Design review of the part built by this model. Coordinates are the model's own, in mm. A direction names the side the tool comes from. Coordinates: 2 decimals unless noted, no trailing zeros. Loops run counter-clockwise (first coordinate to the right, second up) from the corner with the lowest first, then second, coordinate; pieces in that order, holes last. Notation, with made-up numbers: (65.5, -21.5) - (75.5, -21.5) arc R25 cw to (75.5, 6.5) - close; hole circle Ø11 at (-21, 89). An arc over 180 degrees is marked (long way). Use one line per item in the form item = value. Start each with the question number.
(1) The part is to be moulded in two halves that separate along Y. For faces 1 (the face through (0, -10, 9)), 2 (the face through (-35, 65, 9)), 3 (the face through (-20, 25, 9)), say which applies: pulls with the +Y half, pulls with the -Y half, needs draft (parallel to the pull), parting line crosses it, or undercut.
(2) Add section C-C (z = 11). State the section outline as (x, y) points.
(3) Tool access review of faces 4 (the face through (-15, 67, 18)), 5 (the face through (10, 41, 9)): name each direction out of +Z, -Z, +X, -X, +Y, -Y from which nothing blocks a thin tool from reaching the whole face with its end or side.
(4) Add section A-A (x = 0). State the section outline as (y, z) points, plus the area to 3 significant figures.
(5) Add section B-B (y = 56). State the section outline as (x, z) points.
(6) For L1, parallel to X at y = 49, z = 15; L2, parallel to Y at x = -7.5, z = 16.75; L3, parallel to Y at x = 5.5, z = 7.5, list the stretches that pass through material, from the lowest coordinate up.
(7) Clearance check with flat-ended pins moving along their axes: pin 1 Ø3 at (x, z) = (-12, 8) entering from -Y; pin 2 Ø10 at (x, y) = (-3.5, 73) entering from -Z; pin 3 Ø9 at (y, z) = (38.5, 10.5) entering from -X. State where each tip first meets the part, or that it passes through.
Autodesk Inventor part; units mm, degrees
ref_plane "YZ Plane" through (0, 0, 0) normal (1, 0, 0) x (0, 1, 0)
ref_plane "XZ Plane" through (0, 0, 0) normal (0, 1, 0) x (-1, 0, 0)
ref_plane "XY Plane" through (0, 0, 0) normal (0, 0, 1) x (1, 0, 0)
sketch "Sketch1" plane through (0, 0, 0) normal (0, 0, 1) x (1, 0, 0)
  line L0 (0, 0) -> (0, 80) construction
  line L1 (0, 80) -> (10, 80) construction
  line L2 (0, 80) -> (-10, 80) construction
  line L3 (-10, 80) -> (10, 80)
  line L4 (10, 80) -> (10, 0)
  line L5 (-10, 80) -> (-10, 0)
  arc A0 (-10, 0) -> (10, 0) centre (0, 0) ccw
  line L6 (10, 0) -> (20, 0) construction
  line L7 (20, 0) -> (20, 120)
  line L8 (20, 120) -> (-50, 120)
  line L9 (-50, 120) -> (-50, 80)
  line L10 (-50, 120) -> (-20, 120) construction
  arc A1 (-20, 0) -> (20, 0) centre (0, 0) ccw
  line L11 (-20, 0) -> (-20, 50)
  line L12 (-20, 50) -> (-50, 80)
  dimension "d0" = 80
  dimension "d3" = 10
  dimension "d4" = 120
  dimension "d5" = 70
  dimension "d6" = 40
  dimension "d7" = 30
  dimension "d8" = 20
  dimension "d9" = 50
extrude "Extrusion1" add sketch "Sketch1" along normal blind 18
properties part number "guide_3DPrint"
Computed values:
q1.face_1 = undercut
q1.face_2 = pulls with the -Y half
q1.face_3 = needs draft
q2.outline = (-50, 80) - (-20, 50) - (-20, 0) arc R20 ccw to (20, 0) - (20, 120) - (-50, 120) - close; hole (-10, 0) arc R10 ccw to (10, 0) - (10, 80) - (-10, 80) - close
q3.face_4 = +Z, +X, -X, +Y, -Y
q3.face_5 = +Z, -Z
q4.outline = (-20, 0) - (-10, 0) - (-10, 18) - (-20, 18) - close; (80, 0) - (120, 0) - (120, 18) - (80, 18) - close
q4.area = 900 mm^2
q5.outline = (-26, 0) - (-10, 0) - (-10, 18) - (-26, 18) - close; (10, 0) - (20, 0) - (20, 18) - (10, 18) - close
q6.L1 = -20 to -10, 10 to 20
q6.L2 = -18.54 to -6.61, 80 to 120
q6.L3 = -19.23 to -8.35, 80 to 120
q7.pin_1 = -17.02
q7.pin_2 = through
q7.pin_3 = -20
